from build123d import *

# Parameters (mm, degrees)
SKETCH1_W                      = 40
SKETCH1_H                      = 17.8
BOSS_EXTRUDE1_DEPTH            = 3.8
F_5_6_5_6_DIAMETER_HOLE1_D     = 5.6
F_5_6_5_6_DIAMETER_HOLE1_DEPTH = 3.8
FILLET1_R                      = 0.2


with BuildPart() as part:
    # Sketch1 → Boss-Extrude1 (new body)
    with BuildSketch(Plane(origin=(0, 1.9, 0), x_dir=(1, 0, 0), z_dir=(0, 1, 0))):
        Rectangle(SKETCH1_W, SKETCH1_H)
    extrude(amount=-BOSS_EXTRUDE1_DEPTH)

    # Ø5.6 (5.6) Diameter Hole1
    with Locations(Plane(origin=(0, -1.9, 0), x_dir=(-1, 0, 0), z_dir=(0, -1, 0))):
        with Locations((10, 0), (-10, 0)):
            Hole(F_5_6_5_6_DIAMETER_HOLE1_D / 2, depth=F_5_6_5_6_DIAMETER_HOLE1_DEPTH)

    # Fillet1
    fillet1_edges = [part.edges().sort_by_distance(p)[0] for p in [
        (0, -1.9, -8.9),
        (0, -1.9, 8.9),
        (0, 1.9, -8.9),
        (0, 1.9, 8.9),
    ]]
    fillet(fillet1_edges, radius=FILLET1_R)


solid = part.part
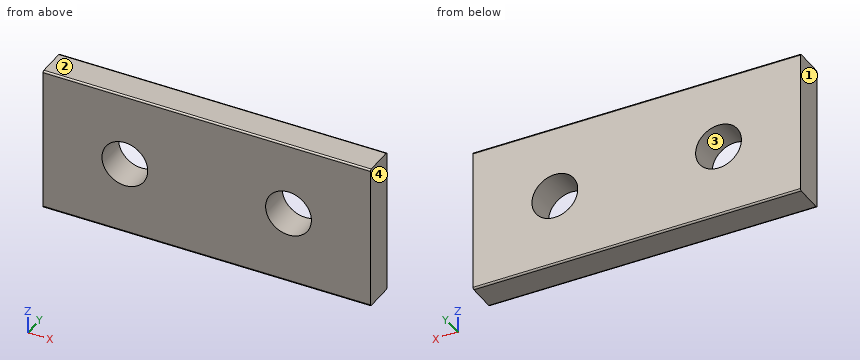
The listing builds one solid part. Answer for the finished solid, in the listing's coordinates (mm). Face numbers are marked on the shaded views. Coordinates: 2 decimals unless noted, no trailing zeros. Loops run counter-clockwise (first coordinate to the right, second up) from the corner with the lowest first, then second, coordinate; pieces in that order, holes last.
1) A flat-ended cylindrical pin translates along its axis: pin 1 Ø5 at (x, z) = (10, 0) entering from +Y. Find the tip coordinate at first contact, or state that the pin passes through.
2) Find section D-D on x = -10.5. Write down the section's boundary in (y, z) (3 decimals).
3) Find section C-C on y = -0.4. Write down the section's boundary in (x, z).
4) Find section B-B on x = 10. Write down the section's boundary in (y, z).
5) Determine the mould class of the marked faces 1, 2, 3 and 4 for opening direction X: pulls with the +X half, pulls with the -X half, needs draft (parallel to the pull), parting line crosses it, or undercut.
6) Find section A-A on z = 0. Write down the section's boundary in (x, y), then the cut area to 3 significant figures.
7) Find the intervals of material crossed by L1, parallel to Z at x = -10, y = -0.35; L2, parallel to X at y = -0.35, z = -2.25; L3, parallel to Z at x = 12.5, y = -1.35, in increasing order.
Values:
1. pin 1: passes through
2. outline: (-1.9, -8.7) arc R0.2 ccw to (-1.7, -8.9) - (1.7, -8.9) arc R0.2 ccw to (1.9, -8.7) - (1.9, -2.755) - (-1.9, -2.755) - close; (-1.9, 2.755) - (1.9, 2.755) - (1.9, 8.7) arc R0.2 ccw to (1.7, 8.9) - (-1.7, 8.9) arc R0.2 ccw to (-1.9, 8.7) - close
3. outline: (-20, -8.9) - (20, -8.9) - (20, 8.9) - (-20, 8.9) - close; hole circle Ø5.6 at (-10, 0); hole circle Ø5.6 at (10, 0)
4. outline: (-1.9, -8.7) arc R0.2 ccw to (-1.7, -8.9) - (1.7, -8.9) arc R0.2 ccw to (1.9, -8.7) - (1.9, -2.8) - (-1.9, -2.8) - close; (-1.9, 2.8) - (1.9, 2.8) - (1.9, 8.7) arc R0.2 ccw to (1.7, 8.9) - (-1.7, 8.9) arc R0.2 ccw to (-1.9, 8.7) - close
5. face 1: pulls with the -X half
5. face 2: needs draft
5. face 3: undercut
5. face 4: pulls with the +X half
6. outline: (-20, -1.9) - (-12.8, -1.9) - (-12.8, 1.9) - (-20, 1.9) - close; (-7.2, -1.9) - (7.2, -1.9) - (7.2, 1.9) - (-7.2, 1.9) - close; (12.8, -1.9) - (20, -1.9) - (20, 1.9) - (12.8, 1.9) - close
6. area: 109 mm2
7. L1: z = -8.9 to -2.8, 2.8 to 8.9
7. L2: x = -20 to -11.67, -8.33 to 8.33, 11.67 to 20
7. L3: z = -8.9 to -1.26, 1.26 to 8.9
